```python
from build123d import *

# Parameters (mm, degrees)
SKETCH1_R             = 15
SKETCH1_R_2           = 10
BOSS_EXTRUDE1_DEPTH   = 15
BOSS_EXTRUDE1_2_DEPTH = 15
SKETCH1_R_3           = 30
SKETCH1_R_4           = 5
SKETCH1_R_5           = 8
BOSS_EXTRUDE1_3_DEPTH = 15
BOSS_EXTRUDE2_DEPTH   = 10


with BuildPart() as part:
    # Sketch1 → Boss-Extrude1 (new, symmetric)
    with BuildSketch(Plane.XY):
        with Locations((-40, -70)):
            Circle(SKETCH1_R)
        with Locations((-40, -70)):
            Circle(SKETCH1_R_2, mode=Mode.SUBTRACT)
    extrude(amount=BOSS_EXTRUDE1_DEPTH, both=True)



with BuildPart() as body_2:
    # Sketch1 → Boss-Extrude1 2 (new, symmetric)
    with BuildSketch(Plane.XY):
        with Locations((40, -70)):
            Circle(SKETCH1_R)
        with Locations((40, -70)):
            Circle(SKETCH1_R_2, mode=Mode.SUBTRACT)
    extrude(amount=BOSS_EXTRUDE1_2_DEPTH, both=True)


with BuildPart() as body_3:
    # Sketch1 → Boss-Extrude1 3 (new, symmetric)
    with BuildSketch(Plane.XY):
        Circle(SKETCH1_R_3)
        with Locations((20, 0)):
            Circle(SKETCH1_R_4, mode=Mode.SUBTRACT)
        with Locations((0, -20)):
            Circle(SKETCH1_R_4, mode=Mode.SUBTRACT)
        with Locations((-20, 0)):
            Circle(SKETCH1_R_4, mode=Mode.SUBTRACT)
        with Locations((0, 20)):
            Circle(SKETCH1_R_4, mode=Mode.SUBTRACT)
        Circle(SKETCH1_R_5, mode=Mode.SUBTRACT)
    extrude(amount=BOSS_EXTRUDE1_3_DEPTH, both=True)


with BuildPart() as part_1:
    add(part.part)

    add(body_2.part)  # Boss-Extrude2 merges body 2

    add(body_3.part)  # Boss-Extrude2 merges body 3
    # Sketch1_3 → Boss-Extrude2 (add, symmetric)
    with BuildSketch(Plane.XY):
        with BuildLine():
            ThreePointArc((30, 0), (0, -30), (-30, 0))
            Line((-30, 0), (-54.061288709, -64.776958756))
            ThreePointArc((-54.061288709, -64.776958756), (-37.3466371, -55.236542908), (-25, -70))
            ThreePointArc((-25, -70), (-26.866074463, -77.245688373), (-32, -82.68857754))
            ThreePointArc((-32, -82.68857754), (0, -73.442887702), (32, -82.68857754))
            ThreePointArc((32, -82.68857754), (30.545301323, -58.354886307), (54.061288709, -64.776958756))
            Line((54.061288709, -64.776958756), (30, 0))
        make_face()
    extrude(amount=BOSS_EXTRUDE2_DEPTH, both=True)


solid = part_1.part
```
CAD build for the part. Positions are in the model's coordinates, mm. A direction names the side the tool comes from. Give positions to 0.01 mm unless a question says otherwise; leave off trailing zeros. Order: outer loops, then holes, each group sorted by start corner. A loop starts at its lowest first (then second) coordinate and runs counter-clockwise, first axis right, second up.
(1) Saw through at A-A, the plane z = 11.5. State how many separate pieces and enclosed holes the cut face has, then the cut area to 3 significant figures.
(2) Tool access for faces 1 (the flat face through (-1, -50, 10)), 2 (the cylindrical face through (-1.08, -24.88, -0.21)): list every direction of +Z, -Z, +X, -X, +Y, -Y with a clear straight run to the whole face (end or side of a thin tool).
(3) Drill centre lines: L1, parallel to Y at x = 0.5, z = -13.25; L2, parallel to X at y = -1.5, z = -7.75; L3, parallel to Y at x = 24, z = 8. Where is each one in solid material? Low to high.
(4) Mould opens along Y. For faces 3 (the cylindrical face through (37.83, -79.76, -0.21)), 4 (the flat face through (50, -73, 15)), 5 (the flat face through (-41.862, -31.935, 0.14)) say: released by +Y, released by -Y, zero draft, split by the parting line, or undercut.
(5) Saw through at C-C, the plane x = 21.5. Give the cut face in (y, z).
(6) Saw through at B-B, the plane z = -3.25. Give the cut face in (x, y).
(7) Flat gauge pins, fed straight in: pin 1 (2 mm diameter, centred on y = 7.5, z = -10, fed in from +X); pin 2 (12 mm diameter, centred on x = 1, z = -10, fed in from -Y); pin 3 (12 mm diameter, centred on x = -29, z = 11.5, fed in from -Y); pin 4 (8 mm diameter, centred on x = 0, y = 20, fed in from +Z) (1 decimal). Where does each tip first touch, or does it go through?
(8) Saw through at D-D, the plane y = -20. Give the cut face in (x, z), then the cut area to 3 significant figures.
Results found:
1. separate pieces: 3
1. enclosed holes: 7
1. area: 3,100 mm2
2. face 1: +Z
2. face 2: +Z, -Z
3. L1: y = -30 to -24.97, -15.03 to -7.98, 7.98 to 15.03, 24.97 to 30
3. L2: x = -30.56 to -24.77, -15.23 to -7.86, 7.86 to 15.23, 24.77 to 30.56
3. L3: y = -78.45 to -3, 3 to 18
4. face 3: undercut
4. face 4: zero draft
4. face 5: released by +Y
5. outline: (-77.43, -10) - (-20.92, -10) - (-20.92, -15) - (-4.77, -15) - (-4.77, 15) - (-20.92, 15) - (-20.92, 10) - (-77.43, 10) - close; (4.77, -15) - (20.92, -15) - (20.92, 15) - (4.77, 15) - close
6. outline: (-54.06, -64.78) arc R15 ccw to (-32, -82.69) arc R60 cw to (32, -82.69) arc R15 ccw to (54.06, -64.78) - (30, 0) arc R30 ccw to (-30, 0) - close; hole circle Ø20 at (-40, -70); hole circle Ø10 at (-20, 0); hole circle Ø16 at (0, 0); hole circle Ø10 at (0, -20); hole circle Ø10 at (0, 20); hole circle Ø10 at (20, 0); hole circle Ø20 at (40, -70)
7. pin 1: stops at x = 29.29
7. pin 2: stops at y = -73.85
7. pin 3: stops at y = -84.14
7. pin 4: passes through
8. outline: (-37.43, -10) - (-22.36, -10) - (-22.36, -15) - (-5, -15) - (-5, 15) - (-22.36, 15) - (-22.36, 10) - (-37.43, 10) - close; (5, -15) - (22.36, -15) - (22.36, -10) - (37.43, -10) - (37.43, 10) - (22.36, 10) - (22.36, 15) - (5, 15) - close
8. area: 1,640 mm2
